```python
from build123d import *

# Parameters (mm, degrees)
F1_DEPTH = 19.05
F2_W     = 44.45
F2_H     = 19.05
F3_DEPTH = 63.5
F5_DEPTH = 44.45
F7_DEPTH = 25.4


with BuildPart() as f1:
    # F0 (on Right) → F1 (new body)
    with BuildSketch(Plane.YZ):
        Polygon((-44.772066, -13.848902), (-44.772066, -26.548902), (18.727934, -26.548902), (18.727934, 17.901098), (-0.322066, 17.436433), align=None)
    extrude(amount=-F1_DEPTH)

    # F2 (on face) → F3 (join)
    with BuildSketch(Plane.YZ):
        with Locations((-3.497066, -17.023902)):
            Rectangle(F2_W, F2_H)
    extrude(amount=F3_DEPTH)

    # F4 (on face) → F5 (join)
    with BuildSketch(Plane(origin=(0, 0, -26.548902), x_dir=(1, 0, 0), z_dir=(0, 0, -1))):
        Polygon((63.5, 25.722066), (63.5, -18.727934), (82.55, -18.727934), (82.55, 44.772066), (63.5, 44.772066), align=None)
    extrude(amount=-F5_DEPTH)

    # F6 (on face) → F7 (cut)
    with BuildSketch(Plane.YZ.offset(82.55)):
        Polygon((-44.772066, 17.901098), (-44.772066, -13.848902), (-0.322066, 17.901098), align=None)
    extrude(amount=-F7_DEPTH, mode=Mode.SUBTRACT)


solid = f1.part
```
Geometry: final body of the model. Coordinates: model frame, mm. A direction names the side the tool comes from. Coordinates: 2 decimals unless noted, no trailing zeros. Order: outer loops, then holes, each group sorted by start corner. A loop starts at its lowest first (then second) coordinate and runs counter-clockwise, first axis right, second up. Notation, with made-up numbers: M 63,6.25 L 78,6.25 A22 ccw 78,30.25 Z; hole C -22.75,8 d8. An arc over 180 degrees is marked long. Answer as CSV lines item,"result".
Q1. Section B-B on x = -6. Return the cut outline in (y, z).
Answers:
outline,"M -44.77,-26.55 L 18.73,-26.55 L 18.73,17.9 L -0.32,17.44 L -44.77,-13.85 Z"
Q2. Section A-A on z = -2. Return the cut outline in (x, y), and give its area (3 significant figures).
Answers:
outline,"M -19.05,-27.94 L 0,-27.94 L 0,18.73 L -19.05,18.73 Z; M 63.5,-28.18 L 82.55,-28.18 L 82.55,18.73 L 63.5,18.73 Z"
area,"1,780 mm^2"
Q3. Draft query along X for faces 1 (the flat face through (-9.39, -22.24, 2.01)), 2 (the flat face through (82.55, -6, -10)), 3 (the flat face through (31, -4, -7.499)). Return one class per face: pulls with the +X half, pulls with the -X half, needs draft (parallel to the pull), parting line crosses it, or undercut.
Answers:
face 1,"needs draft"
face 2,"pulls with the +X half"
face 3,"undercut"
Q4. First-contact query: P1, Ø2, axis at x = 16, y = -20.5, coming from the +Z side; P2, Ø6, axis at x = 13, z = -13, coming from the -Y side; P3, Ø1.5, axis at x = -0.5, y = -23.5, coming from the +Z side. Flat tips, straight axial feed; report the tip coordinate or a pass-through.
Answers:
P1,"stops at z = -7.5"
P2,"stops at y = -25.72"
P3,"stops at z = 1.65"
Q5. Section C-C on y = -33.5. Return the cut outline in (x, z), and give its area (3 significant figures).
Answers:
outline,"M -19.05,-26.55 L 0,-26.55 L 0,-5.92 L -19.05,-5.92 Z; M 63.5,-26.55 L 82.55,-26.55 L 82.55,-5.8 L 63.5,-5.8 Z"
area,"788 mm^2"
Q6. Line query: probe 1 along X at (y, z) = (12.5, 5); probe 2 along Z at (x, y) = (25, -21); probe 3 along Y at (x, z) = (16, -15). Output: solid intervals per line, ascending. Write a range as [from, to].
Answers:
probe 1,"x = [-19.05, 0], [63.5, 82.55]"
probe 2,"z = [-26.55, -7.5]"
probe 3,"y = [-25.72, 18.73]"
Q7. Set-up query: faces 4 (the flat face through (73, -44.772, -20)), 5 (the flat face through (31, -25.722, -17)), 6 (the flat face through (0, -13, -4)). Return all of +Z, -Z, +X, -X, +Y, -Y with unobstructed straight access to the full face (end or side cutting, diameter ignored); none if empty.
Answers:
face 4,"+Z, -Z, +X, -X, -Y"
face 5,"+Z, -Z, -Y"
face 6,"+Z, -Y"
Q8. Section D-D on y = 13. Return the cut outline in (x, z).
Answers:
outline,"M -19.05,-26.55 L 82.55,-26.55 L 82.55,17.9 L 63.5,17.9 L 63.5,-7.5 L 0,-7.5 L 0,17.76 L -19.05,17.76 Z"
